Solid Edge part; units mm, degrees
sketch "Sketch1" plane through (0, 0, 0) normal (0, 0, 1) x (1, 0, 0)
  line L0 (-10, -60) -> (0, -60)
  line L1 (0, -60) -> (0, 0)
  line L2 (0, 0) -> (-42.4264, 42.4264)
  line L3 (-42.4264, 42.4264) -> (-49.4975, 35.3553)
  line L4 (-49.4975, 35.3553) -> (-10, -4.1421)
  line L5 (-10, -4.1421) -> (-10, -60)
  dimension "D1" = 10
  dimension "D2" = 42.4264
extrude "Extrusionsausprägung_3" add sketch "Sketch1" along normal blind 11.5
sketch "Sketch2" plane through (-24.7487, -3.7868, 11.5) normal (0, 0, 1) x (0.7071, -0.7071, 0)
  circle A0 centre (-35.1777, 15.1777) radius 2.5
  circle A1 centre (-5.1777, 15.1777) radius 2.5
extrude "Cutout1" cut sketch "Sketch2" against normal up to next
sketch "Sketch3" plane through (-10, -32.0711, 5) normal (-1, 0, 0) x (0, 1, 0)
  circle A0 centre (-3.9289, 1) radius 1
  circle A1 centre (-22.9289, 1) radius 1
  dimension "D1" = 22.9289
  dimension "D2" = 22.9289
extrude "Cutout2" cut sketch "Sketch3" against normal up to next
properties material "Nylon, allgemein"
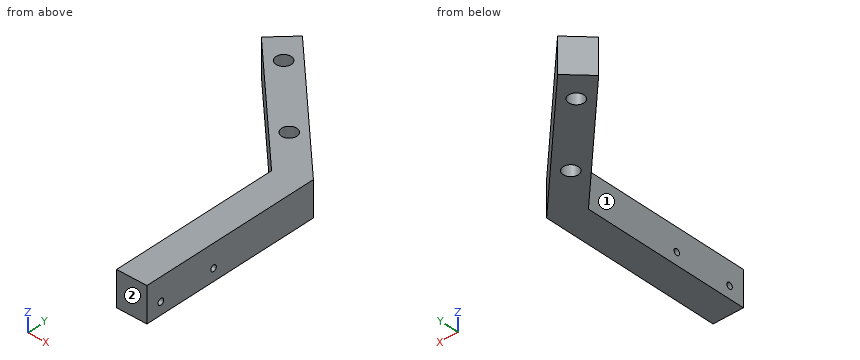
The model under review builds one solid part; all positions refer to its coordinate system, in mm. Face numbers are marked on the shaded views. A direction names the side the tool comes from. Give positions to 0.01 mm unless a question says otherwise; leave off trailing zeros. Write each loop counter-clockwise with the first axis right and the second up, starting at its lowest first coordinate (ties: lowest second). Pieces come first, ordered by that corner, then holes. Notation, with made-up numbers: M 87.25,-15.5 L 117.25,-15.5 A14 ccw 117.25,-2.5 Z; hole C 50,52.5 d1. An arc over 180 degrees is marked long. One line per question, with ' | ' between items. Start each with the question number.
Item 1: Wall thickness on line 1 (Y direction, x = -7.75, z = 4); line 2 (Z direction, x = -3.75, y = -55); line 3 (Y direction, x = -7.25, z = 4): over which ranges is each line inside the solid? List them lowest first. Write a range as from..to.
Item 2: For the marked faces 1 and 2, list the 3-axis set-ups (+Z, -Z, +X, -X, +Y, -Y) from which the entire face can be reached by the end or side of a thin tool; tool diameter is ignored.
Item 3: We need section D-D on z = 9.5. Write out the cut boundary in (x, y).
Item 4: For pin 1 (3 mm diameter, centred on y = 24.5, z = 8.5, fed in from -X); pin 2 (5 mm diameter, centred on y = 11.5, z = 7.5, fed in from -X); pin 3 (6 mm diameter, centred on x = -27.5, z = 9.5, fed in from -Y), all flat-tipped, find the tip position at first contact; note any pin that passes through.
Item 5: We need section B-B on x = -5.5. Write out the cut boundary in (y, z).
Item 6: We need section A-A on y = -55. Write out the cut boundary in (x, z), plus the area to 3 significant figures.
Item 7: We need section C-C on z = 4. Write out the cut boundary in (x, y), plus the area to 3 significant figures.
Results found:
1) line 1: y = -60..-56, -54..-37, -35..7.75 | line 2: z = 0..3, 5..11.5 | line 3: y = -60..-56, -54..-37, -35..7.25
2) face 1: +Z, -Z, -X, -Y | face 2: +Z, -Z, +X, -X, -Y
3) outline: M -49.5,35.36 L -10,-4.14 L -10,-60 L 0,-60 L 0,0 L -42.43,42.43 Z; hole C -38.89,31.82 d5; hole C -17.68,10.61 d5
4) pin 1: stops at x = -40.14 | pin 2: stops at x = -28.14 | pin 3: stops at y = 10.36
5) outline: M -60,0 L 5.5,0 L 5.5,11.5 L -60,11.5 Z; hole C -55,4 d2; hole C -36,4 d2
6) outline: M -10,0 L 0,0 L 0,3 L -10,3 Z; M -10,5 L 0,5 L 0,11.5 L -10,11.5 Z | area: 95.0 mm2
7) outline: M -49.5,35.36 L -10,-4.14 L -10,-35 L 0,-35 L 0,0 L -42.43,42.43 Z; M -10,-60 L 0,-60 L 0,-56 L -10,-56 Z; M -10,-54 L 0,-54 L 0,-37 L -10,-37 Z; hole C -38.89,31.82 d5; hole C -17.68,10.61 d5 | area: 1,080 mm2
